```python
from build123d import *

# Parameters (mm, degrees)
BOSS_EXTRUDE1_START     = -17
BOSS_EXTRUDE1_OUTLINE_W = 38
BOSS_EXTRUDE1_OUTLINE_H = 17
BOSS_EXTRUDE1_DEPTH     = 20
BOSS_EXTRUDE1_2_DEPTH   = 3
BOSS_EXTRUDE1_START_2   = 3
BOSS_EXTRUDE1_3_DEPTH   = 17
BOSS_EXTRUDE1_START_3   = -19
BOSS_EXTRUDE1_4_DEPTH   = 38
SKETCH2_W               = 20
SKETCH2_H               = 38
BOSS_EXTRUDE2_DEPTH     = 3
F_10_CLEARANCE_HOLE1_D  = 5.5
F_10_CLEARANCE_HOLE2_D  = 5.5
F_10_CLEARANCE_HOLE3_D  = 5.5
F_10_CLEARANCE_HOLE4_D  = 5.5
FILLET1_R               = 1


with BuildPart() as part:
    # Boss-Extrude1: read off the stored shape, not the designer's step
    # Boss-Extrude1 outline → Boss-Extrude1 (new body)
    with BuildSketch(Plane.ZY.offset(-3).offset(BOSS_EXTRUDE1_START)):
        with Locations((0, 11.5)):
            Rectangle(BOSS_EXTRUDE1_OUTLINE_W, BOSS_EXTRUDE1_OUTLINE_H)
        with BuildLine():
            ThreePointArc((-15.967743378, 9.378679656), (-10, 16), (-4.032256622, 9.378679656))
            ThreePointArc((-4.032256622, 9.378679656), (-10, 4), (-15.967743378, 9.378679656))
        make_face(mode=Mode.SUBTRACT)
        with BuildLine():
            ThreePointArc((4.032256622, 9.378679656), (10, 16), (15.967743378, 9.378679656))
            ThreePointArc((15.967743378, 9.378679656), (10, 4), (4.032256622, 9.378679656))
        make_face(mode=Mode.SUBTRACT)
    extrude(amount=BOSS_EXTRUDE1_DEPTH)

    # Boss-Extrude1 2 outline → Boss-Extrude1 2 (add)
    with BuildSketch(Plane.ZY.offset(-3)):
        with BuildLine():
            ThreePointArc((4.032256622, 9.378679656), (10, 4), (15.967743378, 9.378679656))
            ThreePointArc((15.967743378, 9.378679656), (10, 16), (4.032256622, 9.378679656))
        make_face()
        with BuildLine():
            ThreePointArc((-15.967743378, 9.378679656), (-10, 4), (-4.032256622, 9.378679656))
            ThreePointArc((-4.032256622, 9.378679656), (-10, 16), (-15.967743378, 9.378679656))
        make_face()
    extrude(amount=BOSS_EXTRUDE1_2_DEPTH)

    # Boss-Extrude1 3 outline → Boss-Extrude1 3 (cut)
    with BuildSketch(Plane(origin=(0, 0, 0), x_dir=(1, 0, 0), z_dir=(0, 1, 0)).offset(BOSS_EXTRUDE1_START_2)):
        with BuildLine():
            ThreePointArc((9.378679656, -15.967743378), (16, -10), (9.378679656, -4.032256622))
            ThreePointArc((9.378679656, -4.032256622), (4, -10), (9.378679656, -15.967743378))
        make_face()
        with BuildLine():
            ThreePointArc((9.378679656, 4.032256622), (16, 10), (9.378679656, 15.967743378))
            ThreePointArc((9.378679656, 15.967743378), (4, 10), (9.378679656, 4.032256622))
        make_face()
    extrude(amount=BOSS_EXTRUDE1_3_DEPTH, mode=Mode.SUBTRACT)

    # Boss-Extrude1 4 outline → Boss-Extrude1 4 (cut)
    with BuildSketch(Plane.XY.offset(BOSS_EXTRUDE1_START_3)):
        Polygon((3, 3), (15.757359313, 3), (3, 15.757359313), align=None)
        Polygon((3, 20), (20, 3), (20, 20), align=None)
    extrude(amount=BOSS_EXTRUDE1_4_DEPTH, mode=Mode.SUBTRACT)

    # Sketch2 → Boss-Extrude2 (add)
    with BuildSketch(Plane.XZ.offset(-3)):
        with Locations((10, 0)):
            Rectangle(SKETCH2_W, SKETCH2_H)
    extrude(amount=BOSS_EXTRUDE2_DEPTH)

    # #10 Clearance Hole1 (through all)
    with Locations(Plane(origin=(0, 3, 0), x_dir=(1, 0, 0), z_dir=(0, 1, 0))):
        with Locations((10, -10)):
            Hole(F_10_CLEARANCE_HOLE1_D / 2)

    # #10 Clearance Hole2 (through all)
    with Locations(Plane.ZY):
        with Locations((-10, 10)):
            Hole(F_10_CLEARANCE_HOLE2_D / 2)

    # #10 Clearance Hole3 (through all)
    with Locations(Plane.ZY):
        with Locations((10, 10)):
            Hole(F_10_CLEARANCE_HOLE3_D / 2)

    # #10 Clearance Hole4 (through all)
    with Locations(Plane(origin=(0, 0, 0), x_dir=(-1, 0, 0), z_dir=(0, -1, 0))):
        with Locations((-10, 10)):
            Hole(F_10_CLEARANCE_HOLE4_D / 2)

    # Fillet1
    fillet1_edges = [part.edges().sort_by_distance(p)[0] for p in [
        (20, 3, 0),
        (3, 20, 0),
    ]]
    fillet(fillet1_edges, radius=FILLET1_R)


solid = part.part
```
Could you check a few things on this model? Use its own coordinates, in mm. A direction names the side the tool comes from. Round coordinates to 2 decimals unless told otherwise and drop trailing zeros. Loops run counter-clockwise (first coordinate to the right, second up) from the corner with the lowest first, then second, coordinate; pieces in that order, holes last. Notation, with made-up numbers: (-16, -3) - (-12, -3) arc R18 ccw to (-12, 12) - close; hole circle Ø2 at (-22, -35). An arc over 180 degrees is marked (long way). Answer in a Markdown table with one row per item. Add a question column.
(1) If we section it at A-A (z = -10): Please give me the cut outline in (x, y), plus the area to 3 significant figures.
(2) If we section it at B-B (y = 5): Please give me the cut outline in (x, z), plus the area to 3 significant figures.
(3) If we mould it in two halves opening along Z, with no side actions, what happens to faces 1 (the face through (20, 1, 0)), 2 (the face through (11.48, 1.52, -12.32)), 3 (the face through (10, 10, 19)), 4 (the face through (1.52, 12.32, 8.52))? For each: pulls with the +Z half, pulls with the -Z half, needs draft (parallel to the pull), parting line crosses it, or undercut.
(4) If we section it at C-C (x = 1.5): Please give me the cut outline in (y, z), plus the area to 3 significant figures.
(5) If we section it at D-D (z = 0): Please give me the cut outline in (x, y), plus the area to 3 significant figures.
(6) I need wall thicknesses on line 1 along Z through (x, y) = (10, 1.95); line 2 along X through (y, z) = (2.3, 10); line 3 along X through (y, z) = (9.25, -15). Which ranges of each line are inside material? Lowest first, please.
(7) For faces 5 (the face through (1.52, 12.32, -11.48)), 6 (the face through (3.7, 16, -10)), 7 (the face through (16, 3.6, 10)), which set-ups out of +Z, -Z, +X, -X, +Y, -Y let a thin tool reach every point of the face, with its end or its side?
(8) I'm going to push flat-ended pins straight in: pin 1 (9.5 mm diameter, centred on y = 10, z = -10, fed in from +X); pin 2 (8 mm diameter, centred on y = 13, z = 14, fed in from +X); pin 3 (3.5 mm diameter, centred on y = 10, z = 10, fed in from +X); pin 4 (4 mm diameter, centred on x = 7, z = 0.5, fed in from +Y). Where does each tip first touch, or does it pass through?
Model answer:
| question | item | result |
|---|---|---|
| 1 | outline | (0, 0) - (7.25, 0) - (7.25, 3) - (3, 3) - (3, 7.25) - (0, 7.25) - close; (0, 12.75) - (3, 12.75) - (3, 16) - (4, 16) - (4, 19) - (3.29, 19.71) arc R1 ccw to (2.59, 20) - (0, 20) - close; (12.75, 0) - (20, 0) - (20, 2.59) arc R1 ccw to (19.71, 3.29) - (19, 4) - (16, 4) - (16, 3) - (12.75, 3) - close |
| 1 | area | 85.0 mm² |
| 2 | outline | (0, -19) - (3, -19) - (3, 19) - (0, 19) - close; (13.76, -19) - (18, -19) - (18, -13.32) - (15, -13.32) arc R6 cw to (13.76, -14.68) - close; (13.76, -5.32) arc R6 cw to (15, -6.68) - (18, -6.68) - (18, 6.68) - (15, 6.68) arc R6 cw to (13.76, 5.32) - close; (13.76, 14.68) arc R6 cw to (15, 13.32) - (18, 13.32) - (18, 19) - (13.76, 19) - close |
| 2 | area | 215 mm² |
| 3 | face 1 | needs draft |
| 3 | face 2 | undercut |
| 3 | face 3 | pulls with the +Z half |
| 3 | face 4 | undercut |
| 4 | outline | (0, -19) - (20, -19) - (20, 19) - (0, 19) - close; hole circle Ø5.5 at (10, -10); hole circle Ø5.5 at (10, 10) |
| 4 | area | 712 mm² |
| 5 | outline | (0, 0) - (20, 0) - (20, 2.59) arc R1 ccw to (19.71, 3.29) - (3.29, 19.71) arc R1 ccw to (2.59, 20) - (0, 20) - close; hole (3, 3) - (15.76, 3) - (3, 15.76) - close |
| 5 | area | 174 mm² |
| 6 | line 1 | z = -19 to -12.75, -7.25 to 7.25, 12.75 to 19 |
| 6 | line 2 | x = 0 to 7.25, 12.75 to 20 |
| 6 | line 3 | x = 0 to 3 |
| 7 | face 5 | +X, -X |
| 7 | face 6 | +X |
| 7 | face 7 | +Y |
| 8 | pin 1 | stops at x = 3 |
| 8 | pin 2 | stops at x = 13.47 |
| 8 | pin 3 | passes through |
| 8 | pin 4 | stops at y = 18 |
